Model file for the job. Use its own axes, mm. Round coordinates to 2 decimals unless told otherwise and drop trailing zeros. Order: outer loops, then holes, each group sorted by start corner. A loop starts at its lowest first (then second) coordinate and runs counter-clockwise, first axis right, second up. Notation, with made-up numbers: (55, 75.25) -> (72, 75.25) arc R22 cw to (72, 106.25) -> close; hole circle Ø5 at (31.5, -12). An arc over 180 degrees is marked (long way). Answer as CSV lines item,"result".
```python
from build123d import *

# Parameters (mm, degrees)
F0_W     = 330.2
F0_H     = 152.4
F1_DEPTH = 12.7
F2_R     = 3.175
F3_DEPTH = 25.4


with BuildPart() as f1:
    # F0 (on Front) → F1 (new body)
    with BuildSketch(Plane.XZ):
        with Locations((5.4142102599, -16.3802644663)):
            Rectangle(F0_W, F0_H)
    extrude(amount=F1_DEPTH)

    # F2 (on face) → F3 (cut)
    with BuildSketch(Plane.XZ.offset(12.7)):
        with BuildLine():
            ThreePointArc((-70.7857897401, -35.4302644663), (-80.0851494374, -12.9796241636), (-102.5357897401, -3.6802644663))
            ThreePointArc((-102.5357897401, -3.6802644663), (-124.9864300428, -12.9796241636), (-134.2857897401, -35.4302644663))
            ThreePointArc((-134.2857897401, -35.4302644663), (-124.9864300428, -57.8809047689), (-102.5357897401, -67.1802644663))
            ThreePointArc((-102.5357897401, -67.1802644663), (-80.0851494374, -57.8809047689), (-70.7857897401, -35.4302644663))
        make_face()
        with BuildLine():
            ThreePointArc((81.6142102599, -35.4302644663), (90.9135700285, -57.8809048401), (113.3642104613, -67.1802644663))
            ThreePointArc((113.3642104613, -67.1802644663), (135.8148506338, -57.8809046977), (145.1142102599, -35.4302644663))
            ThreePointArc((145.1142102599, -35.4302644663), (135.8453787023, -13.0101938717), (113.4506155848, -3.6803820394))
            ThreePointArc((113.4506155848, -3.6803820394), (113.4074129624, -3.6802938596), (113.3642102599, -3.6802644663))
            ThreePointArc((113.3642102599, -3.6802644663), (90.9135699572, -12.9796241636), (81.6142102599, -35.4302644663))
        make_face()
        with Locations((-76.1955228105, -8.7878816322)):
            Circle(F2_R)
        with Locations((-128.5817733597, -8.500114777)):
            Circle(F2_R)
        with Locations((-129.8018724208, -60.0706152875)):
            Circle(F2_R)
        with Locations((-74.9057844611, -60.0706152875)):
            Circle(F2_R)
        with Locations((87.4046319652, -8.500114777)):
            Circle(F2_R)
        with Locations((139.7908825145, -8.7878816322)):
            Circle(F2_R)
        with Locations((141.0806208638, -60.0706152875)):
            Circle(F2_R)
        with Locations((86.1845329041, -60.0706152875)):
            Circle(F2_R)
    extrude(amount=-F3_DEPTH, mode=Mode.SUBTRACT)


solid = f1.part
```
Q1. Saw through at B-B (z = -43.5). Write the cut outline in (x, y), plus the area to 3 significant figures.
Checks:
outline,"(-159.69, -12.7) -> (-133.24, -12.7) -> (-133.24, 0) -> (-159.69, 0) -> close; (-71.83, -12.7) -> (82.66, -12.7) -> (82.66, 0) -> (-71.83, 0) -> close; (144.07, -12.7) -> (170.51, -12.7) -> (170.51, 0) -> (144.07, 0) -> close"
area,"2,630 mm²"
Q2. Wall check: L1, parallel to X at y = -10.25, z = -35; L2, parallel to X at y = -7.75, z = -25.5; L3, parallel to Z at x = 103, y = -11.75. Give the ranges that are in metal, low to high. Write a range as [from, to].
Checks:
L1,"[-159.69, -134.28], [-70.79, 81.62], [145.11, 170.51]"
L2,"[-159.69, -132.69], [-72.38, 83.21], [143.52, 170.51]"
L3,"[-92.58, -65.44], [-5.42, 59.82]"
Q3. Flat gauge pin, fed straight in: pin 1 (8.5 mm diameter, centred on x = 139.79, z = -8.79, fed in from +Y). Where does the tip first touch, or does it go through?
Checks:
pin 1,"y = 0"
Q4. Saw through at A-A (x = 99). Write the cut outline in (y, z), plus the area to 3 significant figures.
Checks:
outline,"(-12.7, -92.58) -> (0, -92.58) -> (0, -63.75) -> (-12.7, -63.75) -> close; (-12.7, -7.12) -> (0, -7.12) -> (0, 59.82) -> (-12.7, 59.82) -> close"
area,"1,220 mm²"
Q5. Mould opens along X. For faces 1 (the flat face through (3, -12.7, -15)), 2 (the cylindrical face through (-130.49, -6.44, -63.17)), 3 (the flat face through (170.514, -6, -17)), 4 (the cylindrical face through (-73.17, -6.44, -7.83)) say: +X half, -X half, draft (parallel to the pull), parting line (faces both ways), or undercut.
Checks:
face 1,"draft"
face 2,"undercut"
face 3,"+X half"
face 4,"undercut"
Q6. Saw through at C-C (y = -10.75). State how many separate pieces and enclosed holes the cut face has, plus the area to 3 significant figures.
Checks:
separate pieces,"1"
enclosed holes,"10"
area,"43,700 mm²"
